Verification items for the finished model (mm, model axes). Give positions to 0.01 mm unless a question says otherwise; leave off trailing zeros. Order: outer loops, then holes, each group sorted by start corner. A loop starts at its lowest first (then second) coordinate and runs counter-clockwise, first axis right, second up.
(1) Scan lines: L1, parallel to X at y = 282, z = 1; L2, parallel to Y at x = -274, z = 2.25. Record each from-to range of solid material in increasing order.
(2) Sectioned sample at B-B on x = -386. Record the cut outline in (y, z).
(3) Gauge pin test, flat ends, axial feed: pin 1 (3 mm diameter, centred on y = 393.5, z = 3.5, fed in from +X); pin 2 (3 mm diameter, centred on y = 76, z = 4.5, fed in from +X); pin 3 (1.9 mm diameter, centred on x = -435, z = 4.5, fed in from -Y). Record the tip position at first contact, or that the pin passes through.
(4) Sectioned sample at C-C on y = 330. Record the cut outline in (x, z), plus the area to 3 significant figures.
(5) Sectioned sample at A-A on z = 3.25. Record the cut outline in (x, y).
```python
from build123d import *

# Parameters (mm, degrees)
SKETCH1_W                = 215.9
SKETCH1_H                = 457.2
BOSS_EXTRUDE1_DEPTH      = 6.35
CUT_EXTRUDE1_DEPTH       = 1
CUT_EXTRUDE1_DEPTH_BACK  = 7.35
CUT_EXTRUDE2_DEPTH       = 1
CUT_EXTRUDE2_DEPTH_BACK  = 7.35
CUT_EXTRUDE3_DEPTH       = 1
CUT_EXTRUDE3_DEPTH_BACK  = 7.35
CUT_EXTRUDE4_DEPTH       = 1
CUT_EXTRUDE4_DEPTH_BACK  = 7.35
CUT_EXTRUDE6_DEPTH       = 1
CUT_EXTRUDE6_DEPTH_BACK  = 7.35
CUT_EXTRUDE7_DEPTH       = 1
CUT_EXTRUDE7_DEPTH_BACK  = 7.35
CUT_EXTRUDE9_DEPTH       = 1
CUT_EXTRUDE9_DEPTH_BACK  = 7.35
CUT_EXTRUDE12_DEPTH      = 1
CUT_EXTRUDE12_DEPTH_BACK = 7.35
CUT_EXTRUDE13_DEPTH      = 7.35
CUT_EXTRUDE14_DEPTH      = 1
CUT_EXTRUDE14_DEPTH_BACK = 7.35
CUT_EXTRUDE15_DEPTH      = 1
CUT_EXTRUDE15_DEPTH_BACK = 7.35
CUT_EXTRUDE16_DEPTH      = 1
CUT_EXTRUDE16_DEPTH_BACK = 7.35


with BuildPart() as part:
    # Sketch1 → Boss-Extrude1 (new body)
    with BuildSketch(Plane.XY):
        with Locations((-336.112358352, 173.908620123)):
            Rectangle(SKETCH1_W, SKETCH1_H)
    extrude(amount=BOSS_EXTRUDE1_DEPTH)

    # Sketch3 → Cut-Extrude1 (cut, two sides)
    with BuildSketch(Plane.XY.offset(6.35)) as cut_extrude1_sk:
        Polygon((-1442.380242436, -41.991379877), (-444.062358352, -41.991379877), (-367.862358352, -41.991379877), (-367.862358352, -54.691379877), (-367.862358352, -1053.009263961), (-1736.075705676, -2507.15733996), (-2810.59358976, -1496.139455876), align=None)
    extrude(amount=CUT_EXTRUDE1_DEPTH, mode=Mode.SUBTRACT)
    extrude(cut_extrude1_sk.sketch, amount=-CUT_EXTRUDE1_DEPTH_BACK, mode=Mode.SUBTRACT)

    # Sketch4 → Cut-Extrude2 (cut, two sides)
    with BuildSketch(Plane.XY.offset(6.35)) as cut_extrude2_sk:
        Polygon((770.155525732, -41.991379877), (-228.162358352, -41.991379877), (-304.362358352, -41.991379877), (-304.362358352, -54.691379877), (-304.362358352, -1053.009263961), (1063.850988971, -2507.15733996), (2138.368873055, -1496.139455876), align=None)
    extrude(amount=CUT_EXTRUDE2_DEPTH, mode=Mode.SUBTRACT)
    extrude(cut_extrude2_sk.sketch, amount=-CUT_EXTRUDE2_DEPTH_BACK, mode=Mode.SUBTRACT)

    # Sketch5 → Cut-Extrude3 (cut, two sides)
    with BuildSketch(Plane.XY.offset(6.35)) as cut_extrude3_sk:
        Polygon((-1321.857723807, -48.341379877), (-367.862358352, -48.341379877), (-304.362358352, -48.341379877), (649.633007102, -48.341379877), (649.633007102, -1956.332110786), (-1321.857723807, -1956.332110786), align=None)
    extrude(amount=CUT_EXTRUDE3_DEPTH, mode=Mode.SUBTRACT)
    extrude(cut_extrude3_sk.sketch, amount=-CUT_EXTRUDE3_DEPTH_BACK, mode=Mode.SUBTRACT)

    # Sketch6 → Cut-Extrude4 (cut, two sides)
    with BuildSketch(Plane.XY.offset(6.35)) as cut_extrude4_sk:
        Polygon((-1430.972246725, 389.808620123), (-444.062358352, 389.808620123), (-367.862358352, 389.808620123), (-367.862358352, 402.508620123), (-367.862358352, 1389.418508496), (-1719.957069161, 2827.404740722), (-2783.066957534, 1827.79485235), align=None)
    extrude(amount=CUT_EXTRUDE4_DEPTH, mode=Mode.SUBTRACT)
    extrude(cut_extrude4_sk.sketch, amount=-CUT_EXTRUDE4_DEPTH_BACK, mode=Mode.SUBTRACT)

    # Sketch7 → Cut-Extrude6 (cut, two sides)
    with BuildSketch(Plane.XY.offset(6.35)) as cut_extrude6_sk:
        Polygon((758.74753002, 389.808620123), (-228.162358352, 389.808620123), (-304.362358352, 389.808620123), (-304.362358352, 402.508620123), (-304.362358352, 1389.418508496), (1047.732352456, 2827.404740722), (2110.842240829, 1827.79485235), align=None)
    extrude(amount=CUT_EXTRUDE6_DEPTH, mode=Mode.SUBTRACT)
    extrude(cut_extrude6_sk.sketch, amount=-CUT_EXTRUDE6_DEPTH_BACK, mode=Mode.SUBTRACT)

    # Sketch8 → Cut-Extrude7 (cut, two sides)
    with BuildSketch(Plane.XY.offset(6.35)) as cut_extrude7_sk:
        Polygon((637.509607102, 396.158620123), (-304.362358352, 396.158620123), (-367.862358352, 396.158620123), (-1309.734323807, 396.158620123), (-1309.734323807, 2279.902551032), (637.509607102, 2279.902551032), align=None)
    extrude(amount=CUT_EXTRUDE7_DEPTH, mode=Mode.SUBTRACT)
    extrude(cut_extrude7_sk.sketch, amount=-CUT_EXTRUDE7_DEPTH_BACK, mode=Mode.SUBTRACT)

    # Sketch9 → Cut-Extrude9 (cut, two sides)
    with BuildSketch(Plane.XY.offset(6.35)) as cut_extrude9_sk:
        Polygon((-240.862358352, -1017.943060863), (-240.862358352, -41.991379877), (-240.862358352, 116.758620123), (-228.162358352, 116.758620123), (747.789322634, 116.758620123), (2219.450453951, -1165.481704095), (1230.798772964, -2300.183385081), align=None)
    extrude(amount=CUT_EXTRUDE9_DEPTH, mode=Mode.SUBTRACT)
    extrude(cut_extrude9_sk.sketch, amount=-CUT_EXTRUDE9_DEPTH_BACK, mode=Mode.SUBTRACT)

    # Sketch10 → Cut-Extrude12 (cut, two sides)
    with BuildSketch(Plane.XY.offset(6.35)) as cut_extrude12_sk:
        Polygon((-240.862358352, 1365.760301109), (-240.862358352, 389.808620123), (-240.862358352, 231.058620123), (-228.162358352, 231.058620123), (747.789322634, 231.058620123), (2219.450453951, 1513.298944341), (1230.798772964, 2648.000625327), align=None)
    extrude(amount=CUT_EXTRUDE12_DEPTH, mode=Mode.SUBTRACT)
    extrude(cut_extrude12_sk.sketch, amount=-CUT_EXTRUDE12_DEPTH_BACK, mode=Mode.SUBTRACT)

    # Sketch12 → Cut-Extrude13 (cut, through all)
    with BuildSketch(Plane.XY.offset(6.35)):
        Polygon((-234.512358352, 939.558620123), (-234.512358352, 231.058620123), (-234.512358352, 116.758620123), (-234.512358352, -591.741379877), (1182.487641648, -591.741379877), (1182.487641648, 939.558620123), align=None)
    extrude(amount=-CUT_EXTRUDE13_DEPTH, mode=Mode.SUBTRACT)

    # Sketch13 → Cut-Extrude14 (cut, two sides)
    with BuildSketch(Plane.XY.offset(6.35)) as cut_extrude14_sk:
        Polygon((-431.362358352, -1012.66894285), (-431.362358352, -41.991379877), (-431.362358352, 116.758620123), (-444.062358352, 116.758620123), (-1414.739921325, 116.758620123), (-2878.883865855, -1158.052046108), (-1895.506302882, -2287.479609081), align=None)
    extrude(amount=CUT_EXTRUDE14_DEPTH, mode=Mode.SUBTRACT)
    extrude(cut_extrude14_sk.sketch, amount=-CUT_EXTRUDE14_DEPTH_BACK, mode=Mode.SUBTRACT)

    # Sketch14 → Cut-Extrude15 (cut, two sides)
    with BuildSketch(Plane.XY.offset(6.35)) as cut_extrude15_sk:
        Polygon((-431.362358352, 1360.486183096), (-431.362358352, 389.808620123), (-431.362358352, 231.058620123), (-444.062358352, 231.058620123), (-1414.739921325, 231.058620123), (-2878.883865855, 1505.869286354), (-1895.506302882, 2635.296849327), align=None)
    extrude(amount=CUT_EXTRUDE15_DEPTH, mode=Mode.SUBTRACT)
    extrude(cut_extrude15_sk.sketch, amount=-CUT_EXTRUDE15_DEPTH_BACK, mode=Mode.SUBTRACT)

    # Sketch16 → Cut-Extrude16 (cut, two sides)
    with BuildSketch(Plane.XY.offset(6.35)) as cut_extrude16_sk:
        Polygon((-437.712358352, 932.013321967), (-437.712358352, 231.058620123), (-437.712358352, 116.758620123), (-437.712358352, -584.196081721), (-1839.62176204, -584.196081721), (-1839.62176204, 932.013321967), align=None)
    extrude(amount=CUT_EXTRUDE16_DEPTH, mode=Mode.SUBTRACT)
    extrude(cut_extrude16_sk.sketch, amount=-CUT_EXTRUDE16_DEPTH_BACK, mode=Mode.SUBTRACT)


solid = part.part
```
Ans:
1. L1: x = -431.36 to -240.86
1. L2: y = -41.99 to 389.81
2. outline: (-41.99, 0) - (389.81, 0) - (389.81, 6.35) - (-41.99, 6.35) - close
3. pin 1: stops at x = -304.36
3. pin 2: stops at x = -240.86
3. pin 3: stops at y = 116.76
4. outline: (-431.36, 0) - (-240.86, 0) - (-240.86, 6.35) - (-431.36, 6.35) - close
4. area: 1,210 mm2
5. outline: (-437.71, 116.76) - (-431.36, 116.76) - (-431.36, -41.99) - (-367.86, -41.99) - (-367.86, -48.34) - (-304.36, -48.34) - (-304.36, -41.99) - (-240.86, -41.99) - (-240.86, 116.76) - (-234.51, 116.76) - (-234.51, 231.06) - (-240.86, 231.06) - (-240.86, 389.81) - (-304.36, 389.81) - (-304.36, 396.16) - (-367.86, 396.16) - (-367.86, 389.81) - (-431.36, 389.81) - (-431.36, 231.06) - (-437.71, 231.06) - close
